Source: CAD feature listing. Evaluate the final solid. Frame: model axes, mm. Face numbers are marked on the shaded views. A direction names the side the tool comes from. Give positions to 0.01 mm unless a question says otherwise; leave off trailing zeros. Order: outer loops, then holes, each group sorted by start corner. A loop starts at its lowest first (then second) coordinate and runs counter-clockwise, first axis right, second up.
from build123d import *

# Parameters (mm, degrees)
SKETCH_1_R      = 10
EXTRUDE_1_DEPTH = 30
SKETCH_3_R      = 5
EXTRUDE_3_DEPTH = 45
SKETCH_4_R      = 15
EXTRUDE_4_DEPTH = 5


with BuildPart() as part:
    # 草图1 → 凸台-拉伸1 (new body)
    with BuildSketch(Plane(origin=(0, 0, 0), x_dir=(1, 0, 0), z_dir=(0, 1, 0))):
        with Locations(Location((0, 0, 0), (0, 0, 270))):
            Circle(SKETCH_1_R)
    extrude(amount=EXTRUDE_1_DEPTH)

    # 草图3 → 凸台-拉伸3 (add)
    with BuildSketch(Plane(origin=(0, 0, 0), x_dir=(0, 0, -1), z_dir=(1, 0, 0))):
        with Locations((0, 7)):
            Circle(SKETCH_3_R)
    extrude(amount=-EXTRUDE_3_DEPTH)

    # 草图4 → 凸台-拉伸4 (add)
    with BuildSketch(Plane.ZY.offset(45)):
        with Locations((0, 7)):
            Circle(SKETCH_4_R)
    extrude(amount=EXTRUDE_4_DEPTH)


solid = part.part
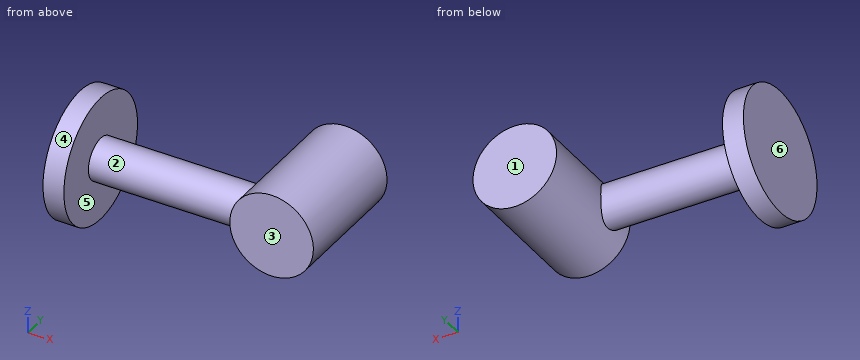
(1) Section A-A, the plane z = 0. Return loops of the section in (x, y), plus the area to 3 significant figures.
(2) Section C-C, the plane y = 7. Return loops of the section in (x, z), plus the area to 4 significant figures.
(3) Section B-B, the plane y = 19. Return loops of the section in (x, z), plus the area to 3 significant figures.
(4) Line query: line 1 along Y through (x, z) = (6.5, 7.5); line 2 along X through (y, z) = (1, -1.75); line 3 along X through (y, z) = (15, -1.5). Output: solid intervals per line, ascending.
(5) Access query for the marked faces 1, 2 and 3. Directions: +Z, -Z, +X, -X, +Y, -Y. A direction counts if a zero-diameter tool reaches every point of the face in a straight line with its end or side. Return the directions, or none.
(6) Draft query along X for the marked faces 4, 5 and 6. Return one class per face: +X half, -X half, draft (parallel to the pull), parting line (faces both ways), or undercut.
(7) Pin query (flat end, axial travel): pin 1 Ø2 at (x, y) = (-6, 5.5) entering from -Z; pin 2 Ø5 at (x, z) = (-16, -0.5) entering from +Y; pin 3 Ø8 at (x, z) = (-35, 4.5) entering from -Y. Return the tip coordinate at first contact, or that it passes through.
(8) Section D-D, the plane x = 0. Return loops of the section in (y, z), plus the area to 3 significant figures.
Checks:
1. outline: (-50, -8) - (-45, -8) - (-45, 2) - (-10, 2) - (-10, 0) - (10, 0) - (10, 30) - (-10, 30) - (-10, 12) - (-45, 12) - (-45, 22) - (-50, 22) - close
1. area: 1,100 mm2
2. outline: (-50, -15) - (-45, -15) - (-45, -5) - (-8.66, -5) arc R10 ccw (long way) to (-8.66, 5) - (-45, 5) - (-45, 15) - (-50, 15) - close
2. area: 818.5 mm2
3. outline: (-50, -9) - (-45, -9) - (-45, 9) - (-50, 9) - close; circle Ø20 at (0, 0)
3. area: 404 mm2
4. line 1: y = 0 to 30
4. line 2: x = -50 to -45, -9.85 to 9.85
4. line 3: x = -50 to -45, -9.89 to 9.89
5. face 1: +Z, -Z, +X, -X, +Y
5. face 2: none
5. face 3: +Z, -Z, +X, -Y
6. face 4: draft
6. face 5: undercut
6. face 6: -X half
7. pin 1: stops at z = -8.66
7. pin 2: stops at y = 12
7. pin 3: stops at y = 2.03
8. outline: (0, -10) - (30, -10) - (30, 10) - (0, 10) - close
8. area: 600 mm2
